from build123d import *

# Parameters (mm, degrees)
F3_R      = 4.5
F4_DEPTH  = 32.5
F8_DEPTH  = 32.5
F6_R      = 4.5
F6_R_2    = 4
F9_DEPTH  = 9
F7_R      = 4.5
F7_R_2    = 4
F10_DEPTH = 11
F11_R     = 2.5
F11_R_2   = 0.75
F12_DEPTH = 4.501


# Not quite as in the source:
# - ends of sketch curves that miss each other by under 0.0002 mm in the source are joined


with BuildPart() as f4:
    # F3 (on Front) → F4 (new body)
    with BuildSketch(Plane.XZ):
        Circle(F3_R)
    extrude(amount=F4_DEPTH)

    # F5 (on face) → F8 (cut, through all)
    with BuildSketch(Plane.XZ.offset(32.5)):
        with BuildLine():
            Line((-1.25, -3.8), (0, -3.8))
            Line((0, -3.8), (1.25, -3.8))
            Line((1.25, -3.8), (1.25, -3.7))
            ThreePointArc((1.25, -3.7), (1.3085786438, -3.5585786438), (1.45, -3.5))
            Line((1.45, -3.5), (2, -3.5))
            Line((2, -3.5), (2, -3.05))
            ThreePointArc((2, -3.05), (2.0585786438, -2.9085786438), (2.2, -2.85))
            Line((2.2, -2.85), (3.15, -2.85))
            Line((3.15, -2.85), (3.15, -2.15))
            Line((3.15, -2.15), (2.2, -2.15))
            ThreePointArc((2.2, -2.15), (2.0585786438, -2.0914213562), (2, -1.95))
            Line((2, -1.95), (2, -1.887459))
            ThreePointArc((2, -1.887459), (2.1033535752, -1.771554046), (2.2, -1.65))
            Line((2.2, -1.65), (3.75, -1.65))
            Line((3.75, -1.65), (3.75, 0))
            Line((3.75, 0), (3.75, 1.65))
            Line((3.75, 1.65), (2.2, 1.65))
            ThreePointArc((2.2, 1.65), (2.1033535752, 1.771554046), (1.9999998047, 1.8874588157))
            Line((1.9999998047, 1.8874588157), (2, 1.95))
            ThreePointArc((2, 1.95), (2.0585786438, 2.0914213562), (2.2, 2.15))
            Line((2.2, 2.15), (3.15, 2.15))
            Line((3.15, 2.15), (3.15, 2.85))
            Line((3.15, 2.85), (2.2, 2.85))
            ThreePointArc((2.2, 2.85), (2.0585786438, 2.9085786438), (2, 3.05))
            Line((2, 3.05), (2, 3.5))
            Line((2, 3.5), (1.45, 3.5))
            ThreePointArc((1.45, 3.5), (1.3085786438, 3.5585786438), (1.25, 3.7))
            Line((1.25, 3.7), (1.25, 3.8))
            Line((1.25, 3.8), (0, 3.8))
            Line((0, 3.8), (-1.25, 3.8))
            Line((-1.25, 3.8), (-1.25, 3.7))
            ThreePointArc((-1.25, 3.7), (-1.3085786438, 3.5585786438), (-1.45, 3.5))
            Line((-1.45, 3.5), (-2, 3.5))
            Line((-2, 3.5), (-2, 3.05))
            ThreePointArc((-2, 3.05), (-2.0585786438, 2.9085786438), (-2.2, 2.85))
            Line((-2.2, 2.85), (-3.15, 2.85))
            Line((-3.15, 2.85), (-3.15, 2.15))
            Line((-3.15, 2.15), (-2.2, 2.15))
            ThreePointArc((-2.2, 2.15), (-2.0585786438, 2.0914213562), (-2, 1.95))
            Line((-2, 1.95), (-2, 1.887459))
            ThreePointArc((-2, 1.887459), (-2.1033535752, 1.771554046), (-2.2, 1.65))
            Line((-2.2, 1.65), (-3.75, 1.65))
            Line((-3.75, 1.65), (-3.75, 0))
            Line((-3.75, 0), (-3.75, -1.65))
            Line((-3.75, -1.65), (-2.2, -1.65))
            ThreePointArc((-2.2, -1.65), (-2.1033535752, -1.771554046), (-1.9999998047, -1.8874588157))
            Line((-1.9999998047, -1.8874588157), (-2, -1.95))
            ThreePointArc((-2, -1.95), (-2.0585786438, -2.0914213562), (-2.2, -2.15))
            Line((-2.2, -2.15), (-3.15, -2.15))
            Line((-3.15, -2.15), (-3.15, -2.85))
            Line((-3.15, -2.85), (-2.2, -2.85))
            ThreePointArc((-2.2, -2.85), (-2.0585786438, -2.9085786438), (-2, -3.05))
            Line((-2, -3.05), (-2, -3.5))
            Line((-2, -3.5), (-1.45, -3.5))
            ThreePointArc((-1.45, -3.5), (-1.3085786438, -3.5585786438), (-1.25, -3.7))
            Line((-1.25, -3.7), (-1.25, -3.8))
        make_face()
    extrude(amount=-F8_DEPTH, mode=Mode.SUBTRACT)

    # F6 (on face) → F9 (join)
    with BuildSketch(Plane.XZ.offset(32.5)):
        Circle(F6_R)
        Circle(F6_R_2, mode=Mode.SUBTRACT)
    extrude(amount=F9_DEPTH)

    # F7 (on face) → F10 (join)
    with BuildSketch(Plane(origin=(0, 0, 0), x_dir=(-1, 0, 0), z_dir=(0, 1, 0))):
        Circle(F7_R)
        Circle(F7_R_2, mode=Mode.SUBTRACT)
    extrude(amount=F10_DEPTH)

    # F11 (on Right) → F12 (cut, through all)
    with BuildSketch(Plane.YZ):
        with Locations((-35.5, 0)):
            Circle(F11_R)
        with Locations((-39.75, 0)):
            Circle(F11_R_2)
    extrude(amount=-F12_DEPTH, mode=Mode.SUBTRACT)


solid = f4.part
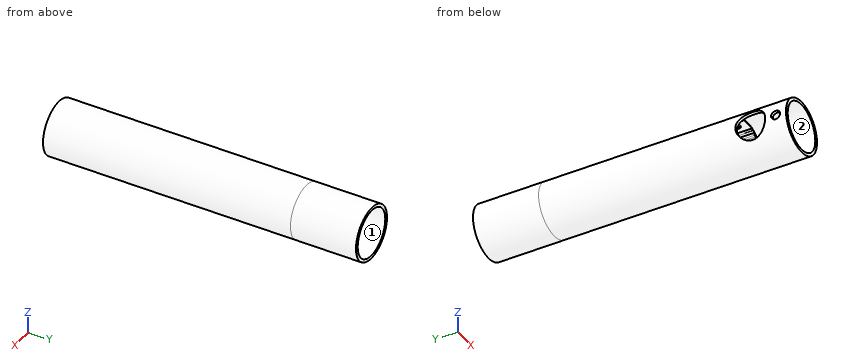
Geometry check sheet. Reference: the model listing, model coordinates, mm. Face numbers are marked on the shaded views. A direction names the side the tool comes from. Round coordinates to 2 decimals unless told otherwise and drop trailing zeros. Order: outer loops, then holes, each group sorted by start corner. A loop starts at its lowest first (then second) coordinate and runs counter-clockwise, first axis right, second up. Notation, with made-up numbers: (60, -29) -> (90, -29) arc R19 ccw to (90, -7) -> close; hole circle Ø5 at (38, -20.75). An arc over 180 degrees is marked (long way). Use one line per item in the form item = value.
1. Go/stop test with flat-tipped pins: pin 1 (5 mm diameter, centred on x = 0.5, z = -0.5, fed in from +Y); pin 2 (2 mm diameter, centred on x = -2, y = -25, fed in from -Z); pin 3 (0.8 mm diameter, centred on x = 3, y = -10, fed in from -Z). Record where each tip stops, or that it passes through.
Working result:
pin_1 = 0
pin_2 = -4.39
pin_3 = -3.67
2. Cross-section at A-A, the plane z = 0. Enter the section's corners in (x, y).
Working result:
outline = (-4.5, -41.5) -> (-4, -41.5) -> (-4, -40.5) -> (-4.5, -40.5) -> close; (-4.5, -39) -> (-4, -39) -> (-4, -38) -> (-4.5, -38) -> close; (-4.5, -33) -> (-4, -33) -> (-4, -32.5) -> (-3.75, -32.5) -> (-3.75, 0) -> (-4, 0) -> (-4, 11) -> (-4.5, 11) -> close; (3.75, -32.5) -> (4, -32.5) -> (4, -41.5) -> (4.5, -41.5) -> (4.5, 11) -> (4, 11) -> (4, 0) -> (3.75, 0) -> close
3. Scan lines: line 1 along Z through (x, y) = (0, -38.25); line 2 along Z through (x, y) = (-2.5, -7); line 3 along Z through (x, y) = (1.5, 3.5). Record each from-to range of solid material in increasing order. Write a range as from..to.
Working result:
line_1 = -4.5..-4, 4..4.5
line_2 = -3.74..-2.85, -2.15..-1.65, 1.65..2.15, 2.85..3.74
line_3 = -4.24..-3.71, 3.71..4.24
4. Set-up check for the marked faces 1 and 2: record each of +Z, -Z, +X, -X, +Y, -Y from which the full face is reachable in a straight line by a thin tool's end or side.
Working result:
face_1 = +Y
face_2 = -Y
5. Cross-section at C-C, the plane y = -35.5. Enter the section's corners in (x, z), plus the area to 3 significant figures.
Working result:
outline = (-3.74, -2.5) arc R4.5 ccw (long way) to (-3.74, 2.5) -> (-3.12, 2.5) arc R4 cw (long way) to (-3.12, -2.5) -> close
area = 10.7 mm^2
6. Cross-section at B-B, the plane x = 0. Enter the section's corners in (y, z), plus the area to 3 significant figures.
Working result:
outline = (-41.5, -4.5) -> (11, -4.5) -> (11, -4) -> (0, -4) -> (0, -3.8) -> (-32.5, -3.8) -> (-32.5, -4) -> (-41.5, -4) -> close; (-41.5, 4) -> (-32.5, 4) -> (-32.5, 3.8) -> (0, 3.8) -> (0, 4) -> (11, 4) -> (11, 4.5) -> (-41.5, 4.5) -> close
area = 65.5 mm^2
